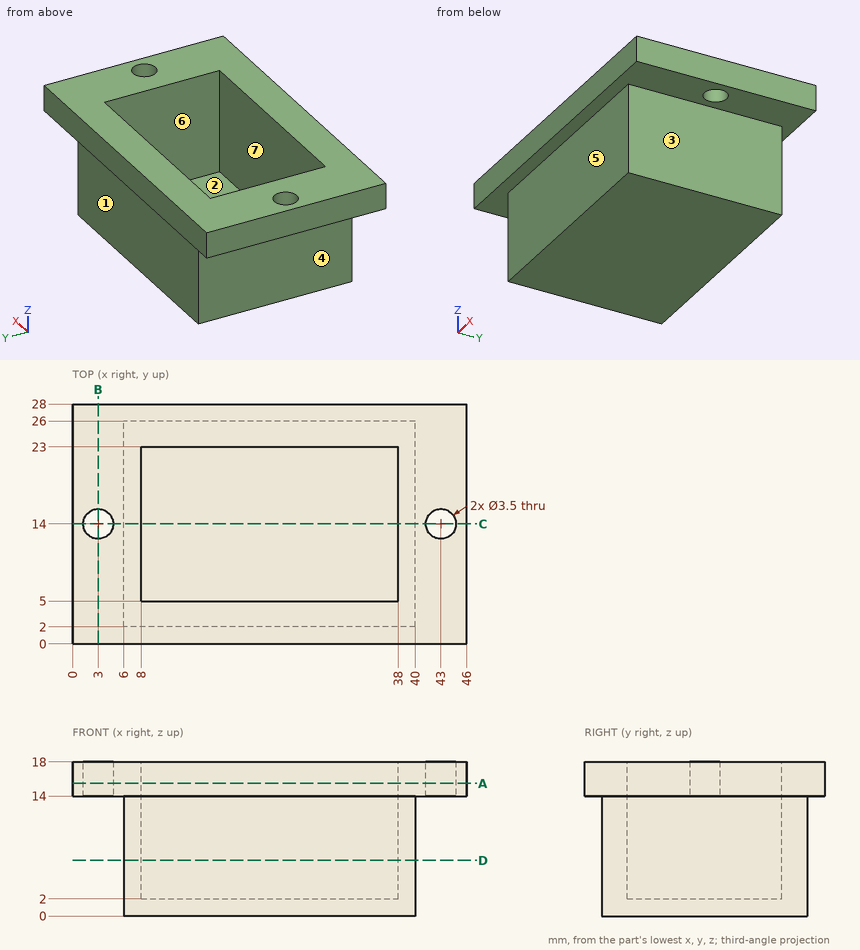
Job drawing, mm, ordinate dimensions from the low corner. One solid piece. A direction names the side the tool comes from. Coordinates: 2 decimals unless noted, no trailing zeros. Order: outer loops, then holes, each group sorted by start corner. A loop starts at its lowest first (then second) coordinate and runs counter-clockwise, first axis right, second up. Notation, with made-up numbers: (4.5, -24) -> (59.5, -24) arc R18 ccw to (59.5, -10) -> close; hole circle Ø1 at (44, 12). An arc over 180 degrees is marked (long way). Answer in a Markdown table with one row per item. Add a question column.
Q1. Band-saw the part on D-D, the plane z = 6.5. List the corners of the cut face in (x, y).
Q2. Band-saw the part on C-C, the plane y = 14. List the corners of the cut face in (x, z).
Q3. Mould opens along Y. For the marked faces 4, 5, 6 and 7 say: +Y half, -Y half, draft (parallel to the pull), parting line (faces both ways), or undercut.
Q4. Wall check: line 1 along Y through (x, z) = (19, 10.5); line 2 along Y through (x, z) = (43, 16.4); line 3 along X through (y, z) = (8.5, 17). Give the ranges that are in metal, low to high. Write a range as [from, to].
Q5. Band-saw the part on B-B, the plane x = 3. List the corners of the cut face in (y, z).
Q6. Drop flat-ended pins along their axis: pin 1 (8 mm diameter, centred on x = 24.5, z = 8, fed in from +Y); pin 2 (1.5 mm diameter, centred on y = 13, z = 13, fed in from +X); pin 3 (1.5 mm diameter, centred on y = 9.5, z = 7, fed in from -X). Give the stop position or say it passes through.
Q7. Band-saw the part on A-A, the plane z = 15.5. List the corners of the cut face in (x, y), then the cut area to 3 significant figures.
Q8. Which spindle directions (+Z, -Z, +X, -X, +Y, -Y) get a long thin tool onto all of the face, cutting with end or side? Do the marked faces 1, 2 and 3. Say none if no direction does.
Answers follow:
| question | item | result |
|---|---|---|
| 1 | outline | (6, 2) -> (40, 2) -> (40, 26) -> (6, 26) -> close; hole (8, 5) -> (38, 5) -> (38, 23) -> (8, 23) -> close |
| 2 | outline | (0, 14) -> (1.25, 14) -> (1.25, 18) -> (0, 18) -> close; (4.75, 14) -> (6, 14) -> (6, 0) -> (40, 0) -> (40, 14) -> (41.25, 14) -> (41.25, 18) -> (38, 18) -> (38, 2) -> (8, 2) -> (8, 18) -> (4.75, 18) -> close; (44.75, 14) -> (46, 14) -> (46, 18) -> (44.75, 18) -> close |
| 3 | face 4 | draft |
| 3 | face 5 | -Y half |
| 3 | face 6 | undercut |
| 3 | face 7 | undercut |
| 4 | line 1 | [2, 5], [23, 26] |
| 4 | line 2 | [0, 12.25], [15.75, 28] |
| 4 | line 3 | [0, 8], [38, 46] |
| 5 | outline | (0, 14) -> (12.25, 14) -> (12.25, 18) -> (0, 18) -> close; (15.75, 14) -> (28, 14) -> (28, 18) -> (15.75, 18) -> close |
| 6 | pin 1 | y = 26 |
| 6 | pin 2 | x = 40 |
| 6 | pin 3 | x = 6 |
| 7 | outline | (0, 0) -> (46, 0) -> (46, 28) -> (0, 28) -> close; hole circle Ø3.5 at (3, 14); hole (8, 5) -> (38, 5) -> (38, 23) -> (8, 23) -> close; hole circle Ø3.5 at (43, 14) |
| 7 | area | 729 mm^2 |
| 8 | face 1 | -Z, +X, -X, +Y |
| 8 | face 2 | +Z |
| 8 | face 3 | -Z, +X, +Y, -Y |
